from build123d import *

# Parameters (mm, degrees)
SKETCH1_W           = 5.08
SKETCH1_H           = 5.08
BOSS_EXTRUDE1_DEPTH = 5.715
SKETCH2_W           = 63.5
SKETCH2_H           = 86.36
BOSS_EXTRUDE2_DEPTH = 5.08
FILLET1_R           = 5.08
SKETCH3_W           = 53.34
SKETCH3_H           = 76.2
BOSS_EXTRUDE3_DEPTH = 3.81
CUT_EXTRUDE1_DEPTH  = 1.27
SKETCH6_W           = 45.72
SKETCH6_H           = 63.5
CUT_EXTRUDE2_DEPTH  = 2.54


with BuildPart() as part:
    # Sketch1 → Boss-Extrude1 (new body)
    with BuildSketch(Plane(origin=(0, 0, 0), x_dir=(1, 0, 0), z_dir=(0, 1, 0))):
        Polygon((-5.08, 0), (0, 0), (0, 76.2), (53.34, 76.2), (53.34, 81.28), (-5.08, 81.28), align=None)
        Polygon((53.34, 0), (0, 0), (0, -5.08), (58.42, -5.08), (58.42, 76.2), (53.34, 76.2), align=None)
        with Locations((-2.54, -2.54)):
            Rectangle(SKETCH1_W, SKETCH1_H)
        with Locations((55.88, 78.74)):
            Rectangle(SKETCH1_W, SKETCH1_H)
    extrude(amount=-BOSS_EXTRUDE1_DEPTH)

    # Sketch2 → Boss-Extrude2 (add)
    with BuildSketch(Plane(origin=(0, -5.715, 0), x_dir=(-1, 0, 0), z_dir=(0, -1, 0))):
        with Locations((-26.67, 38.1)):
            Rectangle(SKETCH2_W, SKETCH2_H)
    extrude(amount=BOSS_EXTRUDE2_DEPTH)

    # Fillet1
    fillet1_edges = [part.edges().sort_by_distance(p)[0] for p in [
        (-5.08, -5.3975, 5.08),
        (-5.08, -5.3975, -81.28),
        (58.42, -5.3975, -81.28),
        (58.42, -5.3975, 5.08),
        (-5.08, -10.795, -38.1),
        (26.67, -10.795, -81.28),
        (58.42, -10.795, -38.1),
        (26.67, -10.795, 5.08),
    ]]
    fillet(fillet1_edges, radius=FILLET1_R)

    # Sketch3 → Boss-Extrude3 (add)
    with BuildSketch(Plane(origin=(0, -5.715, 0), x_dir=(1, 0, 0), z_dir=(0, 1, 0))):
        with Locations((26.67, 38.1)):
            Rectangle(SKETCH3_W, SKETCH3_H)
    extrude(amount=BOSS_EXTRUDE3_DEPTH)

    # Sketch4 → Cut-Extrude1 (cut)
    with BuildSketch(Plane(origin=(0, -1.905, 0), x_dir=(1, 0, 0), z_dir=(0, 1, 0))):
        Polygon((48.895, 69.85), (51.2953, 73.279), (2.0447, 73.279), (4.445, 69.85), align=None)
        Polygon((52.07, 73.279), (51.2953, 73.279), (48.895, 69.85), (49.53, 69.85), (49.53, 6.35), (48.895, 6.35), (51.2953, 2.921), (52.07, 2.921), align=None)
        Polygon((48.895, 6.35), (4.445, 6.35), (2.0447, 2.921), (51.2953, 2.921), align=None)
        Polygon((4.445, 69.85), (2.0447, 73.279), (1.27, 73.279), (1.27, 2.921), (2.0447, 2.921), (4.445, 6.35), (3.81, 6.35), (3.81, 69.85), align=None)
    extrude(amount=-CUT_EXTRUDE1_DEPTH, mode=Mode.SUBTRACT)

    # Sketch6 → Cut-Extrude2 (cut)
    with BuildSketch(Plane(origin=(0, -1.905, 0), x_dir=(1, 0, 0), z_dir=(0, 1, 0))):
        with Locations((26.67, 38.1)):
            Rectangle(SKETCH6_W, SKETCH6_H)
    extrude(amount=-CUT_EXTRUDE2_DEPTH, mode=Mode.SUBTRACT)


solid = part.part
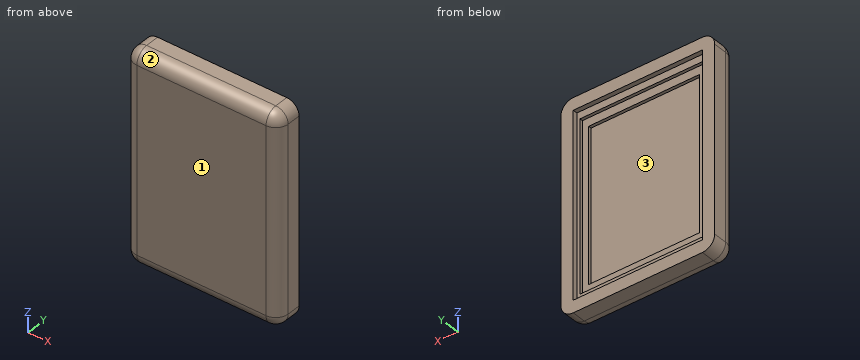
Source: CAD feature listing. Evaluate the final solid. Frame: model axes, mm. Face numbers are marked on the shaded views. Coordinates: 2 decimals unless noted, no trailing zeros. Loops run counter-clockwise (first coordinate to the right, second up) from the corner with the lowest first, then second, coordinate; pieces in that order, holes last. Notation, with made-up numbers: (32.25, 79) - (53.25, 79) arc R22 cw to (53.25, 95) - close; hole circle Ø3 at (77, -39). An arc over 180 degrees is marked (long way). One line per item, written item: value. Start each with the question number.
1. Section D-D (z = -71). Return the cut outline in (x, y) (3 decimals), and give its area (3 significant figures).
2. Section A-A (z = -47). Return the cut outline in (x, y) (3 decimals).
3. Mould query, pull axis Z, two halves, no side actions, for the marked faces 1, 2 and 3. Classes: pulls with the +Z half, pulls with the -Z half, needs draft (parallel to the pull), parting line crosses it, or undercut.
4. Section C-C (y = -7.5). Return the cut outline in (x, z).
5. Section B-B (x = 5). Return the cut outline in (y, z) (3 decimals), and give its area (3 significant figures).
6. Contact query for flat-ended pins moving along their axis: P1, Ø6, axis at y = -8, z = -49.5, coming from the +X side; P2, Ø6, axis at x = 50.5, y = -9.5, coming from the -Z side; P3, Ø5, axis at x = 38.5, y = -8.5, coming from the -Z side; P4, Ø3, axis at x = 19.5, z = -58.5, coming from the +Y side (3 decimals). Output: stop coordinate, or through.
7. Ray query, L1, parallel to Z at x = 17.5, y = -3; L2, parallel to X at y = -3.25, z = -65.5; L3, parallel to Z at x = 23.5, y = -3.25. Return the intervals inside material, ascending.
Verdict:
1. outline: (-5.08, -5.715) arc R5.08 ccw to (0, -10.795) - (53.34, -10.795) arc R5.08 ccw to (58.42, -5.715) - (58.42, 0) - (53.34, 0) - (53.34, -1.905) - (52.07, -1.905) - (52.07, -3.175) - (1.27, -3.175) - (1.27, -1.905) - (0, -1.905) - (0, 0) - (-5.08, 0) - close
1. area: 508 mm2
2. outline: (-5.08, -5.715) arc R5.08 ccw to (0, -10.795) - (53.34, -10.795) arc R5.08 ccw to (58.42, -5.715) - (58.42, 0) - (53.34, 0) - (53.34, -1.905) - (52.07, -1.905) - (52.07, -3.175) - (49.53, -3.175) - (49.53, -4.445) - (3.81, -4.445) - (3.81, -3.175) - (1.27, -3.175) - (1.27, -1.905) - (0, -1.905) - (0, 0) - (-5.08, 0) - close
3. face 1: needs draft
3. face 2: pulls with the +Z half
3. face 3: undercut
4. outline: (-4.76, -76.2) arc R4.76 ccw to (0, -80.96) - (53.34, -80.96) arc R4.76 ccw to (58.1, -76.2) - (58.1, 0) arc R4.76 ccw to (53.34, 4.76) - (0, 4.76) arc R4.76 ccw to (-4.76, 0) - close
5. outline: (-10.795, -76.2) arc R5.08 ccw to (-5.715, -81.28) - (0, -81.28) - (0, -76.2) - (-1.905, -76.2) - (-1.905, -73.279) - (-3.175, -73.279) - (-3.175, -69.85) - (-4.445, -69.85) - (-4.445, -6.35) - (-3.175, -6.35) - (-3.175, -2.921) - (-1.905, -2.921) - (-1.905, 0) - (0, 0) - (0, 5.08) - (-5.715, 5.08) arc R5.08 ccw to (-10.795, 0) - close
5. area: 606 mm2
6. P1: stops at x = 58.42
6. P2: stops at z = -81.22
6. P3: stops at z = -81.27
6. P4: stops at y = -4.445
7. L1: z = -81.28 to -73.28, -2.92 to 5.08
7. L2: x = -5.08 to 3.81, 49.53 to 58.42
7. L3: z = -81.28 to -69.85, -6.35 to 5.08
